Source: CAD feature listing. Evaluate the final solid. Frame: model axes, mm. A direction names the side the tool comes from. Give positions to 0.01 mm unless a question says otherwise; leave off trailing zeros. Loops run counter-clockwise (first coordinate to the right, second up) from the corner with the lowest first, then second, coordinate; pieces in that order, holes last.
```python
from build123d import *

# Parameters (mm, degrees)
SKETCH2_W           = 50.8
SKETCH2_H           = 558.8
BOSS_EXTRUDE1_DEPTH = 50.8
SKETCH5_W           = 50.8
SKETCH5_H           = 50.8
CUT_EXTRUDE1_DEPTH  = 12.7
SKETCH6_W           = 50.8
SKETCH6_H           = 50.8
CUT_EXTRUDE2_DEPTH  = 12.7
SKETCH10_W          = 50.8
SKETCH10_H          = 50.8
CUT_EXTRUDE3_DEPTH  = 12.7
SKETCH11_W          = 50.8
SKETCH11_H          = 50.8
CUT_EXTRUDE4_DEPTH  = 12.7
SKETCH12_R          = 8
CUT_EXTRUDE5_DEPTH  = 16
SKETCH13_R          = 8
CUT_EXTRUDE6_DEPTH  = 16


with BuildPart() as part:
    # Sketch2 → Boss-Extrude1 (new body)
    with BuildSketch(Plane.XY):
        Rectangle(SKETCH2_W, SKETCH2_H)
    extrude(amount=BOSS_EXTRUDE1_DEPTH)

    # Sketch5 → Cut-Extrude1 (cut)
    with BuildSketch(Plane.XY.offset(50.8)):
        with Locations((0, 203.2)):
            Rectangle(SKETCH5_W, SKETCH5_H)
    extrude(amount=-CUT_EXTRUDE1_DEPTH, mode=Mode.SUBTRACT)

    # Sketch6 → Cut-Extrude2 (cut)
    with BuildSketch(Plane(origin=(25.4, 0, 0), x_dir=(0, 0, -1), z_dir=(1, 0, 0))):
        with Locations((-25.4, 203.2)):
            Rectangle(SKETCH6_W, SKETCH6_H)
    extrude(amount=-CUT_EXTRUDE2_DEPTH, mode=Mode.SUBTRACT)

    # Sketch10 → Cut-Extrude3 (cut)
    with BuildSketch(Plane.XY.offset(50.8)):
        with Locations((0, -203.2)):
            Rectangle(SKETCH10_W, SKETCH10_H)
    extrude(amount=-CUT_EXTRUDE3_DEPTH, mode=Mode.SUBTRACT)

    # Sketch11 → Cut-Extrude4 (cut)
    with BuildSketch(Plane(origin=(25.4, 0, 0), x_dir=(0, 0, -1), z_dir=(1, 0, 0))):
        with Locations((-25.4, -203.2)):
            Rectangle(SKETCH11_W, SKETCH11_H)
    extrude(amount=-CUT_EXTRUDE4_DEPTH, mode=Mode.SUBTRACT)

    # Sketch12 → Cut-Extrude5 (cut)
    with BuildSketch(Plane.XZ.offset(279.4)):
        with Locations((0, 25.4)):
            Circle(SKETCH12_R)
    extrude(amount=-CUT_EXTRUDE5_DEPTH, mode=Mode.SUBTRACT)

    # Sketch13 → Cut-Extrude6 (cut)
    with BuildSketch(Plane(origin=(0, 279.4, 0), x_dir=(1, 0, 0), z_dir=(0, 1, 0))):
        with Locations((0, -25.4)):
            Circle(SKETCH13_R)
    extrude(amount=-CUT_EXTRUDE6_DEPTH, mode=Mode.SUBTRACT)


solid = part.part
```
(1) Section B-B, the plane x = 0. Return the cut outline in (y, z), then the cut area to 3 significant figures.
A:
outline: (-279.4, 0) - (279.4, 0) - (279.4, 17.4) - (263.4, 17.4) - (263.4, 33.4) - (279.4, 33.4) - (279.4, 50.8) - (228.6, 50.8) - (228.6, 38.1) - (177.8, 38.1) - (177.8, 50.8) - (-177.8, 50.8) - (-177.8, 38.1) - (-228.6, 38.1) - (-228.6, 50.8) - (-279.4, 50.8) - (-279.4, 33.4) - (-263.4, 33.4) - (-263.4, 17.4) - (-279.4, 17.4) - close
area: 26,600 mm2
(2) First-contact query: pin 1 (9.5 mm diameter, centred on x = 0, z = 25.4, fed in from -Y); pin 2 (13 mm diameter, centred on x = 0, z = 25.4, fed in from +Y); pin 3 (11.5 mm diameter, centred on x = -5.5, y = 194.5, fed in from +Z). Flat tips, straight axial feed; report the tip coordinate or a pass-through.
A:
pin 1: stops at y = -263.4
pin 2: stops at y = 263.4
pin 3: stops at z = 38.1
(3) Mould query, pull axis Z, two halves, no side actions, for faces 1 (the flat face through (-6, -279.4, 19)), 2 (the flat face through (0, 263.4, 25)), 3 (the flat face through (-7, 204, 38.1)). Classes: pulls with the +Z half, pulls with the -Z half, needs draft (parallel to the pull), parting line crosses it, or undercut.
A:
face 1: needs draft
face 2: undercut
face 3: pulls with the +Z half
(4) Section D-D, the plane y = 204.5. Return the cut outline in (x, z), then the cut area to 3 significant figures.
A:
outline: (-25.4, 0) - (12.7, 0) - (12.7, 38.1) - (-25.4, 38.1) - close
area: 1,450 mm2
(5) Section A-A, the plane z = 44.5. Return the cut outline in (x, y), then the cut area to 3 significant figures.
A:
outline: (-25.4, -279.4) - (25.4, -279.4) - (25.4, -228.6) - (-25.4, -228.6) - close; (-25.4, -177.8) - (25.4, -177.8) - (25.4, 177.8) - (-25.4, 177.8) - close; (-25.4, 228.6) - (25.4, 228.6) - (25.4, 279.4) - (-25.4, 279.4) - close
area: 23,200 mm2
(6) Ray query, line 1 along Y through (x, z) = (-20.5, 42); line 2 along Z through (x, y) = (0, -267); line 3 along X through (y, z) = (271.5, 25.4). Return the intervals inside material, ascending.
A:
line 1: y = -279.4 to -228.6, -177.8 to 177.8, 228.6 to 279.4
line 2: z = 0 to 17.4, 33.4 to 50.8
line 3: x = -25.4 to -8, 8 to 25.4
(7) Section C-C, the plane z = 8. Return the cut outline in (x, y), then the cut area to 3 significant figures.
A:
outline: (-25.4, -279.4) - (25.4, -279.4) - (25.4, -228.6) - (12.7, -228.6) - (12.7, -177.8) - (25.4, -177.8) - (25.4, 177.8) - (12.7, 177.8) - (12.7, 228.6) - (25.4, 228.6) - (25.4, 279.4) - (-25.4, 279.4) - close
area: 27,100 mm2
(8) Reachability of faces 4 (the flat face through (11, -177.8, 43)), 5 (the flat face through (0, -263.4, 26)), 6 (the flat face through (0, 254, 50.8)), 7 (the flat face through (-7, -203, 38.1)) from +Z, -Z, +X, -X, +Y, -Y: full face, straight path, thin tool, end or side. Return the list, or none.
A:
face 4: +Z, +X
face 5: -Y
face 6: +Z, +X, -X, +Y, -Y
face 7: +Z, +X, -X
